Geometry: see drawing. Coordinates: mm, zero at the bounding-box minimum. A direction names the side the tool comes from. Give positions to 0.01 mm unless a question says otherwise; leave off trailing zeros. Write each loop counter-clockwise with the first axis right and the second up, starting at its lowest first coordinate (ties: lowest second). Pieces come first, ordered by that corner, then holes. Notation, with made-up numbers: (69.5, 58.5) - (88.5, 58.5) arc R27 cw to (88.5, 88.5) - close; hole circle Ø10 at (33.25, -39). An arc over 180 degrees is marked (long way). Use CSV: the item, a comma, the result in double quotes. Start each with the question number.
(1) Reachability of the marked faces 1 and 2 from +Z, -Z, +X, -X, +Y, -Y: full face, straight path, thin tool, end or side. Return the list, or none.
(2) Section A-A on y = 8. Output: boundary loops of the cut face in (x, z), and give its area (3 significant figures).
(3) Draft query along Y for the marked faces 3, 4 and 5. Return one class per face: released by +Y, released by -Y, zero draft, split by the parting line, or undercut.
(4) First-contact query: pin 1 Ø4 at (y, z) = (14, 39) entering from -X; pin 2 Ø1 at (x, y) = (10.5, 13.5) entering from +Z; pin 3 Ø8 at (x, z) = (2.5, 46.5) entering from +Y. Flat tips, straight axial feed; report the tip coordinate or a pass-through.
(5) Line query: probe 1 along Y at (x, z) = (8, 4.75); probe 2 along Z at (x, y) = (2.25, 12.5); probe 3 along X at (y, z) = (10, 3.5). Output: solid intervals per line, ascending. Write a range as [from, to].
(6) Section D-D on y = 4.5. Output: boundary loops of the cut face in (x, z), and give its area (3 significant figures).
(7) Section B-B on x = 7.25. Output: boundary loops of the cut face in (y, z), and give its area (3 significant figures).
(8) Section C-C on z = 45. Output: boundary loops of the cut face in (x, y).
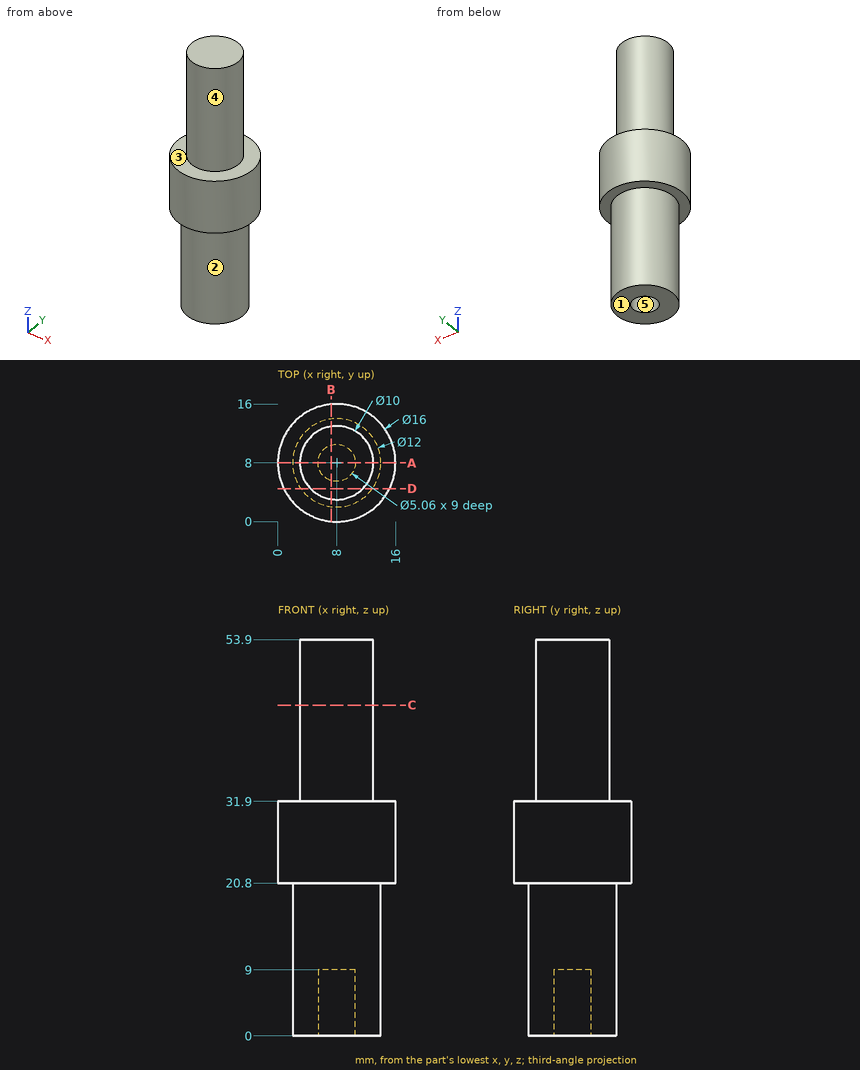
Check values:
1,face 1,"-Z, +X, -X, +Y, -Y"
1,face 2,"-Z"
2,outline,"(0, 20.8) - (2, 20.8) - (2, 0) - (5.47, 0) - (5.47, 9) - (10.53, 9) - (10.53, 0) - (14, 0) - (14, 20.8) - (16, 20.8) - (16, 31.9) - (13, 31.9) - (13, 53.9) - (3, 53.9) - (3, 31.9) - (0, 31.9) - close"
2,area,"602 mm²"
3,face 3,"zero draft"
3,face 4,"split by the parting line"
3,face 5,"undercut"
4,pin 1,"stops at x = 5"
4,pin 2,"stops at z = 31.9"
4,pin 3,"stops at y = 12.77"
5,probe 1,"y = [2, 5.47], [10.53, 14]"
5,probe 2,"z = [20.8, 31.9]"
5,probe 3,"x = [2.34, 6.45], [9.55, 13.66]"
6,outline,"(0.81, 20.8) - (3.13, 20.8) - (3.13, 0) - (12.87, 0) - (12.87, 20.8) - (15.19, 20.8) - (15.19, 31.9) - (11.57, 31.9) - (11.57, 53.9) - (4.43, 53.9) - (4.43, 31.9) - (0.81, 31.9) - close"
6,area,"520 mm²"
7,outline,"(0.04, 20.8) - (2.05, 20.8) - (2.05, 0) - (5.58, 0) - (5.58, 9) - (10.42, 9) - (10.42, 0) - (13.95, 0) - (13.95, 20.8) - (15.96, 20.8) - (15.96, 31.9) - (12.94, 31.9) - (12.94, 53.9) - (3.06, 53.9) - (3.06, 31.9) - (0.04, 31.9) - close"
7,area,"598 mm²"
8,outline,"circle Ø10 at (8, 8)"
